The model under review builds one solid part; all positions refer to its coordinate system, in mm. Round coordinates to 2 decimals unless told otherwise and drop trailing zeros. Write each loop counter-clockwise with the first axis right and the second up, starting at its lowest first coordinate (ties: lowest second). Pieces come first, ordered by that corner, then holes. Notation, with made-up numbers: (18.5, 57.25) -> (77.5, 57.25) arc R20 ccw to (77.5, 78.25) -> close; hole circle Ø4 at (-0.5, 42.25). An arc over 180 degrees is marked (long way). Use CSV: the item, a comma, the result in double quotes. Start each with the question number.
1) Take a section at C-C, the plane y = -0.1. Give the boundary of the cut face in (x, z).
2) Take a section at B-B, the plane x = 43. Give the boundary of the cut face in (y, z), then the cut area to 3 significant figures.
3) For pin 1 Ø3 at (x, z) = (53.4, 13.4) entering from +Y, flat-tipped, find the tip position at first contact; note if it passes through.
4) Take a section at A-A, the plane z = 1. Give the boundary of the cut face in (x, y), then the cut area to 3 significant figures.
5) Wall thickness on probe 1 along X at (y, z) = (-0.8, 13.4); probe 2 along X at (y, z) = (-1.15, -6.5); probe 3 along Z at (x, y) = (-41.5, 0.45): over which ranges is each line inside the solid? List them lowest first. Write a range as [from, to].
from build123d import *

# Parameters (mm, degrees)
SKETCH1_R           = 2.6
BOSS_EXTRUDE1_DEPTH = 1.5
SKETCH2_W           = 7
SKETCH2_H           = 20
CUT_EXTRUDE1_DEPTH  = 64.316664473


with BuildPart() as part:
    # Sketch1 → Boss-Extrude1 (new, symmetric)
    with BuildSketch(Plane(origin=(0, 0, 0), x_dir=(1, 0, 0), z_dir=(0, 1, 0))):
        with BuildLine():
            Line((-53.4, -20), (53.4, -20))
            ThreePointArc((53.4, -20), (58.066904756, -18.066904756), (60, -13.4))
            Line((60, -13.4), (60, 13.4))
            ThreePointArc((60, 13.4), (58.066904756, 18.066904756), (53.4, 20))
            Line((53.4, 20), (-53.4, 20))
            ThreePointArc((-53.4, 20), (-58.066904756, 18.066904756), (-60, 13.4))
            Line((-60, 13.4), (-60, -13.4))
            ThreePointArc((-60, -13.4), (-58.066904756, -18.066904756), (-53.4, -20))
        make_face()
        with Locations(Location((-53.4, 13.4, 0), (0, 0, 270))):
            Circle(SKETCH1_R, mode=Mode.SUBTRACT)
        with Locations(Location((53.4, 13.4, 0), (0, 0, 90))):
            Circle(SKETCH1_R, mode=Mode.SUBTRACT)
        with Locations(Location((53.4, -13.4, 0), (0, 0, 270))):
            Circle(SKETCH1_R, mode=Mode.SUBTRACT)
        with Locations(Location((-53.4, -13.4, 0), (0, 0, 90))):
            Circle(SKETCH1_R, mode=Mode.SUBTRACT)
    extrude(amount=BOSS_EXTRUDE1_DEPTH, both=True)

    # Sketch2 → Cut-Extrude1 (cut, through all)
    with BuildSketch(Plane(origin=(0, 1.5, 0), x_dir=(1, 0, 0), z_dir=(0, 1, 0))):
        with Locations((-41.5, 0)):
            Rectangle(SKETCH2_W, SKETCH2_H)
        with Locations((41.5, 0)):
            Rectangle(SKETCH2_W, SKETCH2_H)
    extrude(amount=-CUT_EXTRUDE1_DEPTH, mode=Mode.SUBTRACT)


solid = part.part
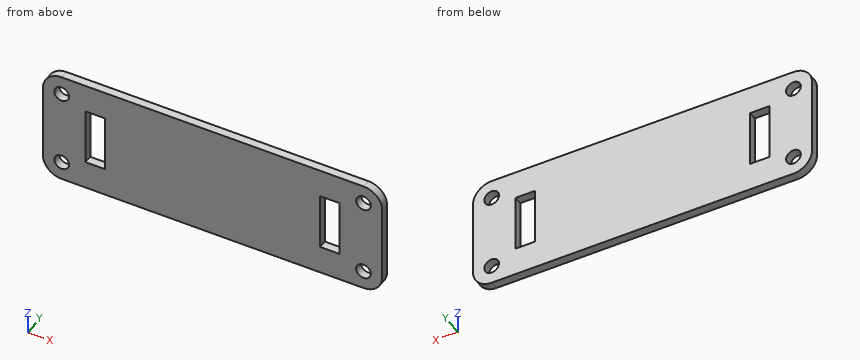
Values found:
1,outline,"(-60, -13.4) arc R6.6 ccw to (-53.4, -20) -> (53.4, -20) arc R6.6 ccw to (60, -13.4) -> (60, 13.4) arc R6.6 ccw to (53.4, 20) -> (-53.4, 20) arc R6.6 ccw to (-60, 13.4) -> close; hole circle Ø5.2 at (-53.4, -13.4); hole circle Ø5.2 at (-53.4, 13.4); hole (-45, -10) -> (-38, -10) -> (-38, 10) -> (-45, 10) -> close; hole (38, -10) -> (45, -10) -> (45, 10) -> (38, 10) -> close; hole circle Ø5.2 at (53.4, -13.4); hole circle Ø5.2 at (53.4, 13.4)"
2,outline,"(-1.5, -20) -> (1.5, -20) -> (1.5, -10) -> (-1.5, -10) -> close; (-1.5, 10) -> (1.5, 10) -> (1.5, 20) -> (-1.5, 20) -> close"
2,area,"60.0 mm²"
3,pin 1,"through"
4,outline,"(-60, -1.5) -> (-45, -1.5) -> (-45, 1.5) -> (-60, 1.5) -> close; (-38, -1.5) -> (38, -1.5) -> (38, 1.5) -> (-38, 1.5) -> close; (45, -1.5) -> (60, -1.5) -> (60, 1.5) -> (45, 1.5) -> close"
4,area,"318 mm²"
5,probe 1,"[-60, -56], [-50.8, 50.8], [56, 60]"
5,probe 2,"[-60, -45], [-38, 38], [45, 60]"
5,probe 3,"[-20, -10], [10, 20]"
